from build123d import *

# Parameters (mm, degrees)
ESQUISSE1_R      = 6.25
EXTRUSION1_DEPTH = 3
ESQUISSE2_R      = 5
EXTRUSION2_DEPTH = 2
ESQUISSE3_R      = 2
EXTRUSION3_DEPTH = 10
CHANFREIN1_SIZE  = 0.5
CHANFREIN2_SIZE  = 0.5
EXTRUSION4_DEPTH = 4


with BuildPart() as part:
    # Esquisse1 → Extrusion1 (new body)
    with BuildSketch(Plane(origin=(0, 0, 0), x_dir=(1, 0, 0), z_dir=(0, 1, 0))):
        Circle(ESQUISSE1_R)
    extrude(amount=EXTRUSION1_DEPTH)

    # Esquisse2 → Extrusion2 (add)
    with BuildSketch(Plane(origin=(0, 3, 0), x_dir=(1, 0, 0), z_dir=(0, 1, 0))):
        Circle(ESQUISSE2_R)
    extrude(amount=EXTRUSION2_DEPTH)

    # Esquisse3 → Extrusion3 (add)
    with BuildSketch(Plane(origin=(0, 5, 0), x_dir=(1, 0, 0), z_dir=(0, 1, 0))):
        Circle(ESQUISSE3_R)
    extrude(amount=EXTRUSION3_DEPTH)

    # Chanfrein1
    chanfrein1_edges = [part.edges().sort_by_distance(p)[0] for p in [
        (-6.25, 0, 0),
        (-6.25, 3, 0),
    ]]
    chamfer(chanfrein1_edges, length=CHANFREIN1_SIZE)

    # Chanfrein2
    chanfrein2_edges = [part.edges().sort_by_distance(p)[0] for p in [
        (-2, 15, 0),
    ]]
    chamfer(chanfrein2_edges, length=CHANFREIN2_SIZE)

    # Esquisse4 → Extrusion4 (cut)
    with BuildSketch(Plane.XZ):
        Polygon((0, 2.309401077), (-2, 1.154700538), (-2, -1.154700538), (0, -2.309401077), (2, -1.154700538), (2, 1.154700538), align=None)
    extrude(amount=-EXTRUSION4_DEPTH, mode=Mode.SUBTRACT)


solid = part.part
Read the model definition and answer for the solid it produces. Units are mm, in the model's axes. A direction names the side the tool comes from. Round coordinates to 2 decimals unless told otherwise and drop trailing zeros. Loops run counter-clockwise (first coordinate to the right, second up) from the corner with the lowest first, then second, coordinate; pieces in that order, holes last. Notation, with made-up numbers: (-36, 40) - (13, 40) arc R25 ccw to (13, 70) - close; hole circle Ø5 at (18.25, 3). An arc over 180 degrees is marked (long way). One line per question, with ' | ' between items. Start each with the question number.
Q1. Find the intervals of material crossed by L1, parallel to Y at x = -4.75, z = -2; L2, parallel to Y at x = -2.25, z = 3.75; L3, parallel to X at y = 2, z = -1.25, in increasing order.
Q2. Section B-B on y = 11 is taken. Give the vertices of the cut face in (x, z).
Q3. Flat-ended cylindrical pins translate along their axes: pin 1 (3 mm diameter, centred on x = -2, y = 8, fed in from +Z); pin 2 (3 mm diameter, centred on x = -4, z = 3.5, fed in from +Y); pin 3 (5 mm diameter, centred on x = 3.5, y = 5, fed in from -Z). Find the tip coordinate at first contact, or state that the pin passes through.
Q4. Section A-A on z = 0 is taken. Give the vertices of the cut face in (x, y).
Q5. For a pull along Z with two mould halves and no side action, classify faces 1 (the cylindrical face through (-1.08, 3.99, 4.88)), 2 (the flat face through (0, 15, 0)), 3 (the flat face through (1.014, 1.972, 1.724)) as +Z half, -Z half, draft (parallel to the pull), parting line (faces both ways), or undercut.
Q6. For faces 4 (the flat face through (0.99, 1.97, -1.74)), 5 (the flat face through (2.5, 0, -0.1)), 6 (the flat face through (-0.1, 5, 2.2)), determine the directions among +Z, -Z, +X, -X, +Y, -Y from which every point of the face is accessible in a straight line to the end or side of a thin tool.
Established:
1) L1: 0 to 3 | L2: 0 to 5 | L3: -6.12 to -1.83, 1.83 to 6.12
2) outline: circle Ø4 at (0, 0)
3) pin 1: z = 1.94 | pin 2: y = 5 | pin 3: z = -5.5
4) outline: (-6.25, 0.5) - (-5.75, 0) - (-2, 0) - (-2, 4) - (2, 4) - (2, 0) - (5.75, 0) - (6.25, 0.5) - (6.25, 2.5) - (5.75, 3) - (5, 3) - (5, 5) - (2, 5) - (2, 14.5) - (1.5, 15) - (-1.5, 15) - (-2, 14.5) - (-2, 5) - (-5, 5) - (-5, 3) - (-5.75, 3) - (-6.25, 2.5) - close
5) face 1: parting line | face 2: draft | face 3: undercut
6) face 4: -Y | face 5: +Z, -Z, +X, -X, -Y | face 6: +Y
